The listing builds one solid part. Answer for the finished solid, in the listing's coordinates (mm). Face numbers are marked on the shaded views. A direction names the side the tool comes from. Coordinates: 2 decimals unless noted, no trailing zeros. Order: outer loops, then holes, each group sorted by start corner. A loop starts at its lowest first (then second) coordinate and runs counter-clockwise, first axis right, second up. Notation, with made-up numbers: (43, 88) - (71, 88) arc R13 ccw to (71, 109) - close; hole circle Ø1 at (65.5, -6). An arc over 180 degrees is marked (long way). Use a Markdown table: item, result. Add a question column.
Item 1: The part is cut by section A-A, the plane x = 0. Give the vertices of the cut face in (y, z) (3 decimals), then the cut area to 3 significant figures.
Item 2: Flat-ended cylindrical pins translate along their axes: P1, Ø4.5, axis at x = 0, y = 27, coming from the +Z side; P2, Ø2, axis at y = 20, z = 5.5, coming from the +X side; P3, Ø3, axis at x = -25, y = 3, coming from the -Z side; P4, Ø2.5, axis at y = 13, z = 1.5, coming from the +X side. Find the tip coordinate at first contact, or state that the pin passes through.
Item 3: The part is cut by section C-C, the plane x = -25. Give the vertices of the cut face in (y, z) (3 decimals).
Item 4: For the marked faces 1 and 2, determine the directions among +Z, -Z, +X, -X, +Y, -Y from which every point of the face is accessible in a straight line to the end or side of a thin tool.
Item 5: The mould has two halves that part along Y. Classify the marked faces 3, 4 and 5: released by +Y, released by -Y, zero draft, split by the parting line, or undercut.
Item 6: The part is cut by section D-D, the plane y = 8.5. Give the vertices of the cut face in (x, z).
Item 7: The part is cut by section B-B, the plane z = 5.5. Give the vertices of the cut face in (x, y).
Item 8: Find the intervals of material crossed by line 1 along X through (y, z) = (27, 1.6); line 2 along Y through (x, z) = (0, 2); line 3 along Y through (x, z) = (-25, 0.85), in increasing order.
from build123d import *

# Parameters (mm, degrees)
BOSS_EXTRUDE1_DEPTH             = 3
M3_CLEARANCE_HOLE1_D            = 3.4
M3_CLEARANCE_HOLE1_CSINK_D      = 3.45
M3_CLEARANCE_HOLE1_CSINK_ANGLE  = 90
SKETCH7_W                       = 3
SKETCH7_H                       = 32
BOSS_EXTRUDE2_DEPTH             = 20
BOSS_EXTRUDE2_DIRECTION_2_REACH = 45.943
M3_CLEARANCE_HOLE2_D            = 3.4
M3_CLEARANCE_HOLE2_CSINK_D      = 3.45
M3_CLEARANCE_HOLE2_CSINK_ANGLE  = 90
FILLET1_R                       = 2
RIB1_REACH                      = 52.45
SKETCH11_WALL_W                 = 114.21465002
SKETCH11_WALL_H                 = 0.75
SKETCH12_R                      = 1.725
CUT_EXTRUDE1_DEPTH              = 50.822183814


with BuildPart() as part:
    # Sketch2 → Boss-Extrude1 (new body)
    with BuildSketch(Plane.XY):
        Polygon((3, 31), (-31, 31), (-31, -1), (3, -1), (3, 8), (-7, 8), (-7, 22), (3, 22), align=None)
    extrude(amount=BOSS_EXTRUDE1_DEPTH)

    # M3 Clearance Hole1 (through all)
    with Locations(Plane(origin=(0, 0, 0), x_dir=(-1, 0, 0), z_dir=(0, 0, -1))):
        with Locations((25, 3), (25, 27), (0, 27), (0, 3)):
            CounterSinkHole(M3_CLEARANCE_HOLE1_D / 2, M3_CLEARANCE_HOLE1_CSINK_D / 2, counter_sink_angle=M3_CLEARANCE_HOLE1_CSINK_ANGLE)

    # Sketch7 → Boss-Extrude2 (add)
    with BuildSketch(Plane.XY.offset(3)):
        with Locations((-30, 15)):
            Rectangle(SKETCH7_W, SKETCH7_H)
    extrude(amount=BOSS_EXTRUDE2_DEPTH)

    # Boss-Extrude2 direction 2: up to this face of the body (flat: up to its plane)
    boss_extrude2_direction_2_end = Plane(part.part.faces().sort_by_distance((-15.906518225, 15, 0))[0])
    # Sketch7 → Boss-Extrude2 direction 2 (add, up to the picked face)
    with BuildSketch(Plane.XY.offset(3), mode=Mode.PRIVATE) as boss_extrude2_direction_2_sk1:
        with Locations((-30, 15)):
            Rectangle(SKETCH7_W, SKETCH7_H)
    boss_extrude2_direction_2_tool1 = split(extrude(boss_extrude2_direction_2_sk1.sketch, amount=-BOSS_EXTRUDE2_DIRECTION_2_REACH, mode=Mode.PRIVATE), bisect_by=boss_extrude2_direction_2_end, keep=Keep.BOTH, mode=Mode.PRIVATE)
    add(boss_extrude2_direction_2_tool1.solids().sort_by(Axis((-30, 15, 3), (0, 0, -1)))[0])

    # M3 Clearance Hole2 (through all)
    with Locations(Plane(origin=(-28.5, 27.5, 0), x_dir=(0, -1, 0), z_dir=(1, 0, 0))):
        with Locations((22.5, -18.5), (2.5, -18.5)):
            CounterSinkHole(M3_CLEARANCE_HOLE2_D / 2, M3_CLEARANCE_HOLE2_CSINK_D / 2, counter_sink_angle=M3_CLEARANCE_HOLE2_CSINK_ANGLE)

    # Fillet1
    fillet1_edges = [part.edges().sort_by_distance(p)[0] for p in [
        (3, 8, 1.5),
        (3, -1, 1.5),
        (3, 31, 1.5),
        (3, 22, 1.5),
        (-30, 31, 23),
        (-30, -1, 23),
    ]]
    fillet(fillet1_edges, radius=FILLET1_R)

    # Sketch11 wall → Rib1 (add, up to next)
    with BuildSketch(Plane(origin=(-24.5, -1, 7), x_dir=(0.707106781187, 0, -0.707106781187), z_dir=(0.707106781187, 0, 0.707106781187)), mode=Mode.PRIVATE) as rib1_sk1:
        with Locations((0, 0.375)):
            Rectangle(SKETCH11_WALL_W, SKETCH11_WALL_H)
    rib1_tool1 = extrude(rib1_sk1.sketch, amount=-RIB1_REACH, mode=Mode.PRIVATE) - part.part
    rib1 = rib1_tool1.solids().sort_by_distance((-24.5, -1, 7))[0]
    add(rib1)

    # Mirror1: Rib1 across plane
    add(rib1.mirror(Plane.ZX.offset(15)))

    # Sketch12 → Cut-Extrude1 (cut, through all)
    with BuildSketch(Plane(origin=(-28.5, 0, 0), x_dir=(0, 0, -1), z_dir=(1, 0, 0))):
        with BuildLine():
            Line((-20.425, 5), (-20.045779221, 4.234368496))
            ThreePointArc((-20.045779221, 4.234368496), (-20.225, 5), (-20.045779221, 5.765631504))
            Line((-20.045779221, 5.765631504), (-20.425, 5))
        make_face()
        with BuildLine():
            ThreePointArc((-16.775, 5), (-16.820402704, 4.606836011), (-16.954220779, 4.234368496))
            Line((-16.954220779, 4.234368496), (-16.575, 5))
            Line((-16.575, 5), (-16.954220779, 5.765631504))
            ThreePointArc((-16.954220779, 5.765631504), (-16.820402704, 5.393163989), (-16.775, 5))
        make_face()
        with BuildLine():
            ThreePointArc((-16.775, 25), (-16.820402704, 24.606836011), (-16.954220779, 24.234368496))
            Line((-16.954220779, 24.234368496), (-16.575, 25))
            Line((-16.575, 25), (-16.954220779, 25.765631504))
            ThreePointArc((-16.954220779, 25.765631504), (-16.820402704, 25.393163989), (-16.775, 25))
        make_face()
        with BuildLine():
            Line((-20.425, 25), (-20.045779221, 24.234368496))
            ThreePointArc((-20.045779221, 24.234368496), (-20.225, 25), (-20.045779221, 25.765631504))
            Line((-20.045779221, 25.765631504), (-20.425, 25))
        make_face()
        with Locations((-18.5, 25)):
            Circle(SKETCH12_R)
        with BuildLine():
            ThreePointArc((-20.045779221, 5.765631504), (-20.225, 5), (-20.045779221, 4.234368496))
            ThreePointArc((-20.045779221, 4.234368496), (-19.409645715, 3.534336439), (-18.5, 3.275))
            Line((-18.5, 3.275), (-18.5, 6.725))
            ThreePointArc((-18.5, 6.725), (-19.409645715, 6.465663561), (-20.045779221, 5.765631504))
        make_face()
        with BuildLine():
            Line((-18.5, 6.725), (-18.5, 3.275))
            ThreePointArc((-18.5, 3.275), (-17.590354285, 3.534336439), (-16.954220779, 4.234368496))
            ThreePointArc((-16.954220779, 4.234368496), (-16.820402704, 4.606836011), (-16.775, 5))
            ThreePointArc((-16.775, 5), (-16.820402704, 5.393163989), (-16.954220779, 5.765631504))
            ThreePointArc((-16.954220779, 5.765631504), (-17.590354285, 6.465663561), (-18.5, 6.725))
        make_face()
    extrude(amount=-CUT_EXTRUDE1_DEPTH, mode=Mode.SUBTRACT)


solid = part.part
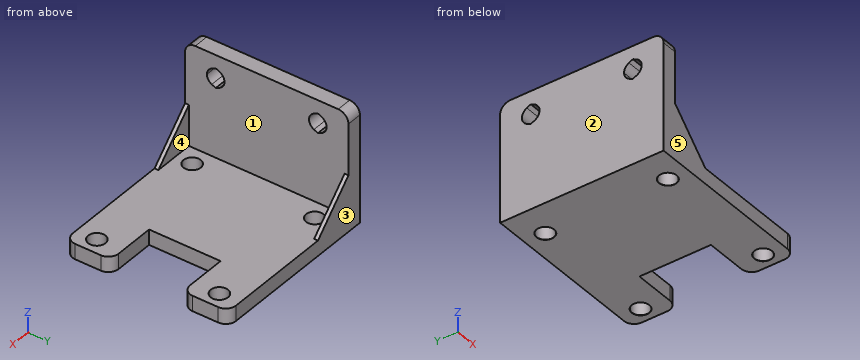
Solution:
| question | item | result |
|---|---|---|
| 1 | outline | (-1, 0) - (1.275, 0) - (1.3, 0.025) - (1.3, 3) - (-1, 3) - close; (4.7, 0.025) - (4.725, 0) - (8, 0) - (8, 3) - (4.7, 3) - close; (22, 0) - (25.275, 0) - (25.3, 0.025) - (25.3, 3) - (22, 3) - close; (28.7, 0.025) - (28.725, 0) - (31, 0) - (31, 3) - (28.7, 3) - close |
| 1 | area | 33.6 mm2 |
| 2 | P1 | stops at z = 3 |
| 2 | P2 | stops at x = -28.5 |
| 2 | P3 | passes through |
| 2 | P4 | stops at x = -7 |
| 3 | outline | (-1, 0) - (1.275, 0) - (1.3, 0.025) - (1.3, 3) - (-0.25, 3) - (-0.25, 7.5) - (-1, 7.5) - close; (4.7, 0.025) - (4.725, 0) - (25.275, 0) - (25.3, 0.025) - (25.3, 3) - (4.7, 3) - close; (28.7, 0.025) - (28.725, 0) - (31, 0) - (31, 7.5) - (30.25, 7.5) - (30.25, 3) - (28.7, 3) - close |
| 4 | face 1 | +Z, +X |
| 4 | face 2 | +Z, -Z, -X, +Y, -Y |
| 5 | face 3 | released by +Y |
| 5 | face 4 | undercut |
| 5 | face 5 | released by -Y |
| 6 | outline | (-31.5, 0) - (-7, 0) - (-7, 3) - (-28.5, 3) - (-28.5, 23) - (-31.5, 23) - close |
| 7 | outline | (-31.5, -1) - (-23, -1) - (-23, -0.25) - (-28.5, -0.25) - (-28.5, 30.25) - (-23, 30.25) - (-23, 31) - (-31.5, 31) - close |
| 8 | line 1 | x = -31.5 to -26.7, -23.3 to -1.7, 1.7 to 3 |
| 8 | line 2 | y = -1 to 1.3, 4.7 to 8, 22 to 25.3, 28.7 to 31 |
| 8 | line 3 | y = -1 to 1.3, 4.7 to 25.3, 28.7 to 31 |
